Can you work these out from the drawing? Everything is in mm from the part's minimum corner. A direction names the side the tool comes from. Give positions to 0.01 mm unless a question says otherwise; leave off trailing zeros. Loops run counter-clockwise (first coordinate to the right, second up) from the corner with the lowest first, then second, coordinate; pieces in that order, holes last. Notation, with made-up numbers: (47.25, 19) - (62.25, 19) arc R17 ccw to (62.25, 37) - close; hole circle Ø9 at (-34.75, -23.5). An arc over 180 degrees is marked (long way). One line per item, written item: value. Start each with the question number.
Q1. If we mould it in two halves opening along X, with no side actions, what happens to the marked faces 1 and 2? For each: released by +X, released by -X, zero draft, split by the parting line, or undercut.
Q2. I'm going to push flat-ended pins straight in: P1, Ø1, axis at x = 6.5, y = 16, coming from the +Z side; P2, Ø3, axis at x = 1, y = 14.5, coming from the +Z side. Where does each tip first touch, or does it pass through?
Q3. I want a section at B-B (x = 4). Please give me the cut outline in (y, z), then the cut area to 3 significant figures.
Q4. I want a section at A-A (z = 4). Please give me the cut outline in (x, y).
Q5. For the marked faces 3 and 4, which set-ups out of +Z, -Z, +X, -X, +Y, -Y let a thin tool reach every point of the face, with its end or its side?
Q6. I want a section at D-D (x = 2). Please give me the cut outline in (y, z), then the cut area to 3 significant figures.
Q7. I want a section at C-C (y = 21). Please give me the cut outline in (x, z).
Q8. If I drill on line 1 (Y direction, x = 3.75, z = 6); line 2 (Y direction, x = 3, z = 1); line 3 (Z direction, x = 4.25, y = 16), over which ranges is the centre line in solid material (lowest first)? Write a range as from..to.
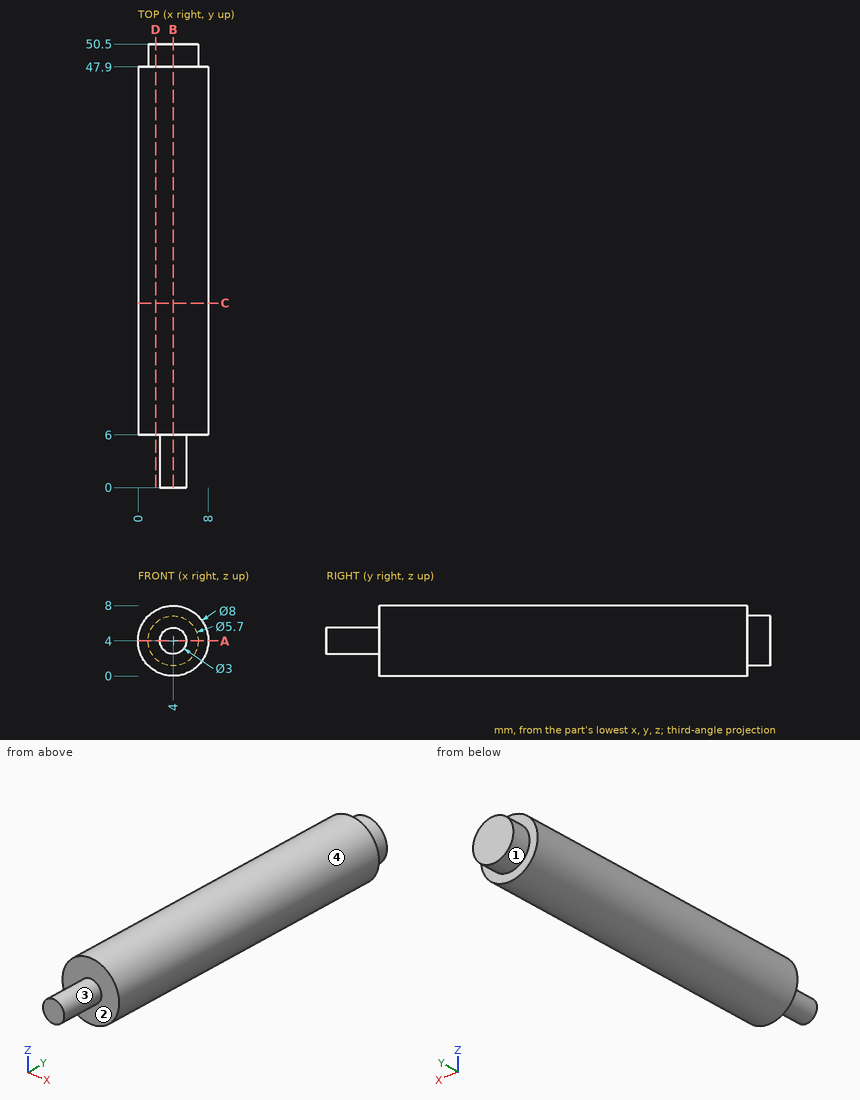
Worked answers:
1. face 1: split by the parting line
1. face 2: zero draft
2. P1: stops at z = 7.46
2. P2: stops at z = 7.71
3. outline: (0, 2.5) - (6, 2.5) - (6, 0) - (47.9, 0) - (47.9, 1.15) - (50.5, 1.15) - (50.5, 6.85) - (47.9, 6.85) - (47.9, 8) - (6, 8) - (6, 5.5) - (0, 5.5) - close
3. area: 368 mm²
4. outline: (0, 6) - (2.5, 6) - (2.5, 0) - (5.5, 0) - (5.5, 6) - (8, 6) - (8, 47.9) - (6.85, 47.9) - (6.85, 50.5) - (1.15, 50.5) - (1.15, 47.9) - (0, 47.9) - close
5. face 3: -Y
5. face 4: +Y, -Y
6. outline: (6, 0.54) - (47.9, 0.54) - (47.9, 1.97) - (50.5, 1.97) - (50.5, 6.03) - (47.9, 6.03) - (47.9, 7.46) - (6, 7.46) - close
6. area: 301 mm²
7. outline: circle Ø8 at (4, 4)
8. line 1: y = 6..50.5
8. line 2: y = 6..47.9
8. line 3: z = 0.01..7.99
